Could you check a few things on this model? Use its own coordinates, in mm. Face numbers are marked on the shaded views. A direction names the side the tool comes from. Give positions to 0.01 mm unless a question says otherwise; leave off trailing zeros. Loops run counter-clockwise (first coordinate to the right, second up) from the corner with the lowest first, then second, coordinate; pieces in that order, holes last. Notation, with made-up numbers: (-20, 17.5) -> (13, 17.5) arc R4 cw to (13, 22.5) -> close; hole circle Ø4 at (8, -38.5). An arc over 180 degrees is marked (long way). Write item = value, one per line. Start each with the question number.
1) I want a section at A-A (z = 84). List the corners of the cut face in (x, y) for me.
2) I want a section at C-C (z = -8.5). List the corners of the cut face in (x, y) for me.
3) If we mould it in two halves opening along X, with no side actions, what happens to the marked faces 3, 4, 5 and 6? For each: +X half, -X half, draft (parallel to the pull), parting line (faces both ways), or undercut.
4) I want a section at D-D (y = 343.5). List the corners of the cut face in (x, z) for me.
5) I want a section at B-B (x = -24). List the corners of the cut face in (y, z) for me, and give its area (3 significant figures).
6) On a 3-axis mill with a long thin cutter (end or side, diameter ignored), from which of +Z, -Z, +X, -X, +Y, -Y can I reach the whole of each face in a straight line? I mean the marked faces 1 and 2. Say none if no direction works.
7) I need wall thicknesses on probe 1 along X at (y, z) = (41.5, 78); probe 2 along Z at (x, y) = (-142, 252.5). Which ranges of each line are inside material? Lowest first, please. Write a range as from..to.
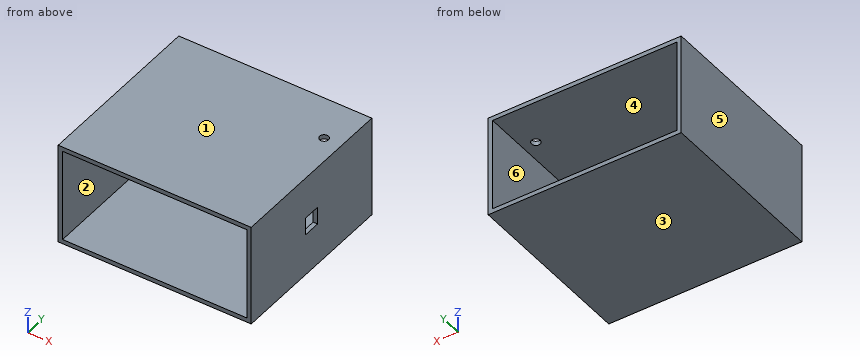
from build123d import *

# Parameters (mm, degrees)
F0_W     = 438.88918
F0_H     = 231.110052
F0_W_2   = 418.88918
F0_H_2   = 211.110052
F1_DEPTH = 400
F3_D     = 20
F3_DEPTH = 12.4
F4_W     = 40
F4_H     = 40
F5_DEPTH = 10


with BuildPart() as f1:
    # F0 (on Front) → F1 (new body)
    with BuildSketch(Plane.XZ):
        Rectangle(F0_W, F0_H)
        Rectangle(F0_W_2, F0_H_2, mode=Mode.SUBTRACT)
    extrude(amount=-F1_DEPTH)

    # F3
    with Locations(Plane.XY.offset(115.555026)):
        with Locations((179.44459, 300)):
            Hole(F3_D / 2, depth=F3_DEPTH)

    # F4 (on face) → F5 (cut, through all)
    with BuildSketch(Plane.YZ.offset(219.44459)):
        with Locations((200, 0)):
            Rectangle(F4_W, F4_H)
    extrude(amount=-F5_DEPTH, mode=Mode.SUBTRACT)


solid = f1.part
Answer list:
q1.outline = (-219.44, 0) -> (-209.44, 0) -> (-209.44, 400) -> (-219.44, 400) -> close; (209.44, 0) -> (219.44, 0) -> (219.44, 400) -> (209.44, 400) -> close
q2.outline = (-219.44, 0) -> (-209.44, 0) -> (-209.44, 400) -> (-219.44, 400) -> close; (209.44, 0) -> (219.44, 0) -> (219.44, 180) -> (209.44, 180) -> close; (209.44, 220) -> (219.44, 220) -> (219.44, 400) -> (209.44, 400) -> close
q3.face_3 = draft
q3.face_4 = undercut
q3.face_5 = -X half
q3.face_6 = undercut
q4.outline = (-219.44, -115.56) -> (219.44, -115.56) -> (219.44, 115.56) -> (-219.44, 115.56) -> close; hole (-209.44, -105.56) -> (209.44, -105.56) -> (209.44, 105.56) -> (-209.44, 105.56) -> close
q5.outline = (0, -115.56) -> (400, -115.56) -> (400, -105.56) -> (0, -105.56) -> close; (0, 105.56) -> (400, 105.56) -> (400, 115.56) -> (0, 115.56) -> close
q5.area = 8,000 mm^2
q6.face_1 = +Z, +X, -X, +Y, -Y
q6.face_2 = +Y, -Y
q7.probe_1 = -219.44..-209.44, 209.44..219.44
q7.probe_2 = -115.56..-105.56, 105.56..115.56
